Autodesk Inventor part; units mm, degrees
ref_plane "YZ Plane" through (0, 0, 0) normal (1, 0, 0) x (0, 1, 0)
ref_plane "XZ Plane" through (0, 0, 0) normal (0, 1, 0) x (-1, 0, 0)
ref_plane "XY Plane" through (0, 0, 0) normal (0, 0, 1) x (1, 0, 0)
sketch "Sketch1" plane through (0, 0, 0) normal (0, 0, 1) x (1, 0, 0)
  line L0 (-490, 68) -> (490, 68)
  line L1 (490, 68) -> (490, 0)
  line L2 (490, 0) -> (-490, 0)
  line L3 (-490, 0) -> (-490, 68)
  point P0 (0, 0)
  point P1 (0, 0)
  dimension "d0" = 980
  dimension "d1" = 68
extrude "Plate1" add sketch "Sketch1" along normal blind 2
sketch "Sketch2" plane through (490, 2, 0) normal (0, -1, 0) x (1, 0, 0)
  line L0 (-980, 0) -> (0, 0)
  line L1 (0, 0) -> (0, 20)
  line L2 (0, 20) -> (-980, 20)
  line L3 (-980, 20) -> (-980, 0)
edge flange "Flange1" height 20 angle 90 thickness 2 bend radius 2.75 thickness toward (0, -1, 0) relief round relief width 2 relief depth 1 edges at (0, 0, 2) wall of the first edge with corners at (-490, 2, 0) (490, 2, 0) (490, 2, 20) (-490, 2, 20)
bend "Bend1"
corner "Corner1"
sketch "Sketch5" plane through (0, 0, 0) normal (0, 0, -1) x (-1, 0, 0)
  line L0 (490, 68) -> (-490, 68)
  line L1 (490, 0) -> (-490, 0)
  circle A0 centre (0, 68) radius 35
  line L2 (243.95, 68) -> (246.05, 68)
  line L3 (246.05, 68) -> (246.05, 27)
  line L4 (246.05, 27) -> (243.95, 27)
  line L5 (243.95, 27) -> (243.95, 68)
  line L6 (-243.95, 68) -> (-246.05, 68)
  line L7 (-246.05, 68) -> (-246.05, 27)
  line L8 (-246.05, 27) -> (-243.95, 27)
  line L9 (-243.95, 27) -> (-243.95, 68)
  line L10 (0, 68) -> (0, 0) construction
  point P0 (0, 0)
  point P1 (245, 27)
  point P2 (-245, 27)
  point P3 (-35, 68)
  point P4 (35, 68)
  dimension "d45" = 70
  dimension "d48" = 2.1
  dimension "d49" = 490
  dimension "d51" = 27
  dimension "d52" = 41
extrude "Extrusion1" cut sketch "Sketch5" against normal through all contours L3 L4 L5 L0 | L9 L8 L7 L0 | A0 L0 picked at (-5.3545, 54.8926)
sketch "Sketch9" plane through (0, 0, 2) normal (0, 0, 1) x (1, 0, 0)
  line L0 (485.6141, 29.596) -> (485.6141, 17.596) construction
  line L1 (485.6141, 17.596) -> (285.6141, 17.596) construction
  line L2 (285.6141, 17.596) -> (285.6141, 29.596) construction
  line L3 (285.6141, 29.596) -> (485.6141, 29.596) construction
  line L4 (-490, 68) -> (490, 68)
  point P0 (0, 0)
  point P1 (1.05, 68)
  dimension "d40" = 200
  dimension "d41" = 12
mark "Mark2"
equation "\"d1\" = СПИНА_Стрингер_2_высота"
equation "\"d2\" = Thickness"
equation "\"d3\" = BendReliefWidth"
equation "\"d4\" = BendReliefDepth"
equation "\"d5\" = MinimumRemnant"
equation "\"d6\" = TransitionRadius"
equation "\"d9\" = BendRadius"
equation "\"d10\" = CornerReliefSize"
equation "\"d11\" = GapSize"
equation "\"d12\" = JacobiRadiusSize"
equation "\"BendReliefWidth\" = Thickness"
equation "\"BendReliefDepth\" = 0.5 * Thickness"
equation "\"CornerReliefSize\" = 4 * Thickness"
equation "\"MinimumRemnant\" = 2 * Thickness"
equation "\"TransitionRadius\" = BendRadius"
equation "\"JacobiRadiusSize\" = BendRadius"
equation "\"GapSize\" = Thickness"
properties part number "MSC 206 STRINGER BACK ^^" material "Stainless Steel"
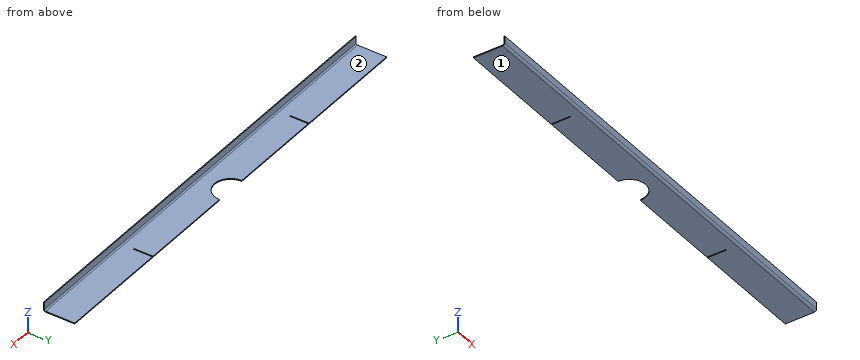
The model under review builds one solid part; all positions refer to its coordinate system, in mm. Face numbers are marked on the shaded views. A direction names the side the tool comes from. Give positions to 0.01 mm unless a question says otherwise; leave off trailing zeros. Loops run counter-clockwise (first coordinate to the right, second up) from the corner with the lowest first, then second, coordinate; pieces in that order, holes last. Notation, with made-up numbers: (86, -16) -> (109, -16) arc R12 cw to (109, -12) -> close; hole circle Ø4 at (34, 53.25). An arc over 180 degrees is marked (long way). Put each result on its own line as item: value. Start each with the question number.
1. We need section A-A on x = 363.5. State the section outline as (y, z) points, then the cut area to 3 significant figures.
2. Clearance check with flat-ended pins moving along their axes: P1, Ø3, axis at x = -384.5, z = 11.5, coming from the +Y side; P2, Ø1, axis at x = -245, z = 1.5, coming from the +Y side; P3, Ø10, axis at x = -337.5, y = 44, coming from the +Z side; P4, Ø1.5, axis at x = -157, y = 48, coming from the -Z side. State where each tip first meets the part, or that it passes through.
3. Wall thickness on probe 1 along X at (y, z) = (44.5, 1.25); probe 2 along X at (y, z) = (62, 1.25); probe 3 along Y at (x, z) = (111.5, 12): over which ranges is each line inside the solid? List them lowest first.
4. We need section D-D on x = 0. State the section outline as (y, z) points, then the cut area to 3 significant figures.
5. For the marked faces 1 and 2, list the 3-axis set-ups (+Z, -Z, +X, -X, +Y, -Y) from which the entire face can be reached by the end or side of a thin tool; tool diameter is ignored.
6. We need section B-B on y = 18. State the section outline as (x, z) points, then the cut area to 3 significant figures.
Determined:
1. outline: (0, 4.75) arc R4.75 ccw to (4.75, 0) -> (68, 0) -> (68, 2) -> (4.75, 2) arc R2.75 cw to (2, 4.75) -> (2, 20) -> (0, 20) -> close
1. area: 169 mm^2
2. P1: y = 2
2. P2: y = 27
2. P3: z = 2
2. P4: z = 0
3. probe 1: -490 to -246.05, -243.95 to -25.94, 25.94 to 243.95, 246.05 to 490
3. probe 2: -490 to -246.05, -243.95 to -34.48, 34.48 to 243.95, 246.05 to 490
3. probe 3: 0 to 2
4. outline: (0, 4.75) arc R4.75 ccw to (4.75, 0) -> (33, 0) -> (33, 2) -> (4.75, 2) arc R2.75 cw to (2, 4.75) -> (2, 20) -> (0, 20) -> close
4. area: 98.8 mm^2
5. face 1: -Z, +X, -X, +Y, -Y
5. face 2: +Z, +X, -X, +Y
6. outline: (-490, 0) -> (490, 0) -> (490, 2) -> (-490, 2) -> close
6. area: 1,960 mm^2
